from build123d import *

# Parameters (mm, degrees)
SKETCH1_R           = 2.6
BOSS_EXTRUDE1_DEPTH = 10
SKETCH1_3_W         = 20
SKETCH1_3_H         = 5
BOSS_EXTRUDE2_DEPTH = 20
SKETCH1_4_R         = 2.6
CUT_EXTRUDE1_DEPTH  = 5.5
SKETCH2_R           = 2
BOSS_EXTRUDE3_DEPTH = 4
FILLET1_R           = 1
FILLET2_R           = 2


with BuildPart() as part:
    # Sketch1 → Boss-Extrude1 (new, symmetric)
    with BuildSketch(Plane.XY):
        with BuildLine():
            Line((-2.686718641, 19.396732815), (-10, 5))
            Line((-10, 5), (10, 5))
            Line((10, 5), (11.424127203, 14.935887565))
            ThreePointArc((11.424127203, 14.935887565), (6.260691915, 23.151172776), (-2.686718641, 19.396732815))
        make_face()
        with Locations((4, 16)):
            Circle(SKETCH1_R, mode=Mode.SUBTRACT)
    extrude(amount=BOSS_EXTRUDE1_DEPTH, both=True)

    # Sketch1<3> → Boss-Extrude2 (add, symmetric)
    with BuildSketch(Plane.XY):
        with Locations((0, 2.5)):
            Rectangle(SKETCH1_3_W, SKETCH1_3_H)
    extrude(amount=BOSS_EXTRUDE2_DEPTH, both=True)

    # Sketch1<4> → Cut-Extrude1 (cut, symmetric)
    with BuildSketch(Plane.XY):
        with BuildLine():
            ThreePointArc((11.424127203, 14.935887565), (6.260691915, 23.151172776), (-2.686718641, 19.396732815))
            Line((-2.686718641, 19.396732815), (-10, 5))
            Line((-10, 5), (10, 5))
            Line((10, 5), (11.424127203, 14.935887565))
        make_face()
        with Locations((4, 16)):
            Circle(SKETCH1_4_R, mode=Mode.SUBTRACT)
    extrude(amount=CUT_EXTRUDE1_DEPTH, both=True, mode=Mode.SUBTRACT)

    # Sketch2 → Boss-Extrude3 (add)
    with BuildSketch(Plane.XZ):
        with Locations(Location((0, 10, 0), (0, 0, 90))):
            Circle(SKETCH2_R)
        with Locations(Location((0, -10, 0), (0, 0, 90))):
            Circle(SKETCH2_R)
    extrude(amount=BOSS_EXTRUDE3_DEPTH)

    # Fillet1
    fillet1_edges = [part.edges().sort_by_distance(p)[0] for p in [
        (-10, 2.5, -20),
        (10, 2.5, 20),
        (-10, 2.5, 20),
        (10, 2.5, -20),
    ]]
    fillet(fillet1_edges, radius=FILLET1_R)

    # Fillet2
    # the kernel refuses this fillet: 2 mm, written as the material it adds along each edge
    with BuildSketch(Plane(origin=(-10, 5, 10), x_dir=(0, 0, 1), z_dir=(1, 0, 0))) as fillet2_piece_1_section:
        with BuildLine():
            CenterArc((FILLET2_R, -FILLET2_R), FILLET2_R, 90, 90)
            Line((0, -FILLET2_R), (0, 0))
            Line((0, 0), (FILLET2_R, 0))
        make_face()
    fillet2_piece_1 = extrude(amount=20, mode=Mode.PRIVATE)
    fillet2_piece_1 = split(fillet2_piece_1, bisect_by=Plane(origin=(-7.744522427, 9.440073667, 10.455584543), z_dir=(0.8915624854306203, -0.45289770872988017, 0)), keep=Keep.TOP, mode=Mode.PRIVATE)
    fillet2_piece_1 = split(fillet2_piece_1, bisect_by=Plane(origin=(9.863918043, 4.050579875, 10.455584543), z_dir=(-0.9898836270660257, 0.14188165796398555, 0)), keep=Keep.TOP, mode=Mode.PRIVATE)
    add(fillet2_piece_1)
    with BuildSketch(Plane(origin=(-10, 5, 10), x_dir=(0, 0, 1), z_dir=(1, 0, 0))) as fillet2_piece_2_section:
        with BuildLine():
            CenterArc((FILLET2_R, -FILLET2_R), FILLET2_R, 90, 90)
            Line((0, -FILLET2_R), (0, 0))
            Line((0, 0), (FILLET2_R, 0))
        make_face()
    fillet2_piece_2 = extrude(amount=25, mode=Mode.PRIVATE)
    fillet2_piece_2 = split(fillet2_piece_2, bisect_by=Plane(origin=(10, 5.860236103, 10.212945025), z_dir=(1, 0, 0)), keep=Keep.TOP, mode=Mode.PRIVATE)
    fillet2_piece_2 = split(fillet2_piece_2, bisect_by=Plane(origin=(10.122058034, 5.851577653, 10.212945025), z_dir=(-0.9898836270660257, 0.14188165796398555, 0)), keep=Keep.TOP, mode=Mode.PRIVATE)
    add(fillet2_piece_2)
    with BuildSketch(Plane(origin=(-10, 5, -10), x_dir=(0, 0, -1), z_dir=(1, 0, 0))) as fillet2_piece_3_section:
        with BuildLine():
            CenterArc((FILLET2_R, FILLET2_R), FILLET2_R, 180, 90)
            Line((0, FILLET2_R), (0, 0))
            Line((0, 0), (FILLET2_R, 0))
        make_face()
    fillet2_piece_3 = extrude(amount=20, mode=Mode.PRIVATE)
    fillet2_piece_3 = split(fillet2_piece_3, bisect_by=Plane(origin=(-7.744522427, 9.440073667, -10.455584543), z_dir=(0.8915624854306203, -0.45289770872988017, 0)), keep=Keep.TOP, mode=Mode.PRIVATE)
    fillet2_piece_3 = split(fillet2_piece_3, bisect_by=Plane(origin=(9.863918043, 4.050579875, -10.455584543), z_dir=(-0.9898836270660257, 0.14188165796398555, 0)), keep=Keep.TOP, mode=Mode.PRIVATE)
    add(fillet2_piece_3)
    with BuildSketch(Plane(origin=(-10, 5, -10), x_dir=(0, 0, -1), z_dir=(1, 0, 0))) as fillet2_piece_4_section:
        with BuildLine():
            CenterArc((FILLET2_R, FILLET2_R), FILLET2_R, 180, 90)
            Line((0, FILLET2_R), (0, 0))
            Line((0, 0), (FILLET2_R, 0))
        make_face()
    fillet2_piece_4 = extrude(amount=25, mode=Mode.PRIVATE)
    fillet2_piece_4 = split(fillet2_piece_4, bisect_by=Plane(origin=(10, 5.860236103, -10.212945025), z_dir=(1, 0, 0)), keep=Keep.TOP, mode=Mode.PRIVATE)
    fillet2_piece_4 = split(fillet2_piece_4, bisect_by=Plane(origin=(10.122058034, 5.851577653, -10.212945025), z_dir=(-0.9898836270660257, 0.14188165796398555, 0)), keep=Keep.TOP, mode=Mode.PRIVATE)
    add(fillet2_piece_4)


solid = part.part
Geometry: final body of the model. Coordinates: model frame, mm. A direction names the side the tool comes from. Coordinates: 2 decimals unless noted, no trailing zeros. Order: outer loops, then holes, each group sorted by start corner. A loop starts at its lowest first (then second) coordinate and runs counter-clockwise, first axis right, second up.
1) Section A-A (x = 4). Return loops of the section in (y, z), then the cut area to 3 significant figures.
Result sheet:
outline: (0, -20) - (5, -20) - (5, -12) arc R2 cw to (7, -10) - (13.4, -10) - (13.4, -5.5) - (5, -5.5) - (5, 5.5) - (13.4, 5.5) - (13.4, 10) - (7, 10) arc R2 cw to (5, 12) - (5, 20) - (0, 20) - close; (18.6, -10) - (23.5, -10) - (23.5, -5.5) - (18.6, -5.5) - close; (18.6, 5.5) - (23.5, 5.5) - (23.5, 10) - (18.6, 10) - close
area: 321 mm2
2) First-contact query: P1, Ø2.5, axis at y = 1.5, z = 4, coming from the +X side; P2, Ø2, axis at x = 5.5, y = 13, coming from the -Z side; P3, Ø2, axis at y = 13, z = 5, coming from the -X side. Flat tips, straight axial feed; report the tip coordinate or a pass-through.
Result sheet:
P1: stops at x = 10
P2: stops at z = -10
P3: stops at x = -6.38
3) Ray query, probe 1 along Z at (x, y) = (2.25, 14); probe 2 along Y at (x, z) = (4, 8.65); probe 3 along Y at (x, z) = (-4.5, 4.5). Return the intervals inside material, ascending.
Result sheet:
probe 1: z = -10 to -5.5, 5.5 to 10
probe 2: y = 0 to 13.4, 18.6 to 23.5
probe 3: y = 0 to 5
4) Section C-C (x = -6.5). Return loops of the section in (y, z).
Result sheet:
outline: (0, -20) - (5, -20) - (5, -12) arc R2 cw to (7, -10) - (11.89, -10) - (11.89, -5.5) - (5, -5.5) - (5, 5.5) - (11.89, 5.5) - (11.89, 10) - (7, 10) arc R2 cw to (5, 12) - (5, 20) - (0, 20) - close
5) Set-up query: faces 4 (the flat face through (0, 5, 0)), 5 (the flat face through (1, 14, -10)), 6 (the flat face through (1, 14, 10)), 7 (the flat face through (10, 3, 0)), 8 (the cylindrical face through (1.2, -2, -11.6)). Return all of +Z, -Z, +X, -X, +Y, -Y with unobstructed straight access to the full face (end or side cutting, diameter ignored); none if empty.
Result sheet:
face 4: +X, -X, +Y
face 5: -Z, +X, -X, +Y
face 6: +Z, +X, -X, +Y
face 7: +Z, -Z, +X, -Y
face 8: -Y
6) Section D-D (y = 14.5). Return loops of the section in (x, z), then the cut area to 3 significant figures.
Result sheet:
outline: (-5.17, -10) - (1.88, -10) - (1.88, -5.5) - (-5.17, -5.5) - close; (-5.17, 5.5) - (1.88, 5.5) - (1.88, 10) - (-5.17, 10) - close; (6.12, -10) - (11.36, -10) - (11.36, -5.5) - (6.12, -5.5) - close; (6.12, 5.5) - (11.36, 5.5) - (11.36, 10) - (6.12, 10) - close
area: 111 mm2
7) Draft query along Z for faces 1 (the cylindrical face through (0, 5.6, -10.57)), 2 (the flat face through (3, 12, -5.5)), 3 (the cylindrical face through (-9.715, 2.535, 19.699)). Return one class per face: released by +Z, released by -Z, zero draft, split by the parting line, or undercut.
Result sheet:
face 1: released by -Z
face 2: undercut
face 3: released by +Z
8) Section B-B (y = -2). Return loops of the section in (x, z).
Result sheet:
outline: circle Ø4 at (0, -10); circle Ø4 at (0, 10)
